```python
from build123d import *

# Parameters (mm, degrees)
F0_W     = 56
F0_H     = 90
F1_DEPTH = 25
F2_DEPTH = 60
F3_SIZE  = 17
F5_D     = 13
F5_DEPTH = 11
F5_TIP   = 3.9055940237
F6_R     = 5


with BuildPart() as f1:
    # F0 (on Top) → F1 (new body)
    with BuildSketch(Plane.XY):
        with Locations((28, 45)):
            Rectangle(F0_W, F0_H)
    extrude(amount=F1_DEPTH)

    # F2 (add): a face of the model
    f2_faces = [f1.faces().sort_by_distance(p)[0] for p in [
        (28, 45, 25),
    ]]
    extrude(f2_faces, amount=F2_DEPTH)

    # F3
    f3_edges = [f1.edges().sort_by_distance(p)[0] for p in [
        (56, 45, 85),
    ]]
    chamfer(f3_edges, length=F3_SIZE)

    # F5
    with Locations(Plane(origin=(62, 0, 62), x_dir=(0, 1, 0), z_dir=(0.7071067812, 0, 0.7071067812))):
        with Locations((20, 20.5269119346), (70, 20.5269119346)):
            Hole(F5_D / 2, depth=F5_DEPTH)
            with Locations((0, 0, -(F5_DEPTH + F5_TIP / 2))):  # 118° drill point
                Cone(0, F5_D / 2, F5_TIP, mode=Mode.SUBTRACT)

    # F6
    f6_edges = [f1.edges().sort_by_distance(p)[0] for p in [
        (28, 0, 0),
        (28, 90, 0),
    ]]
    fillet(f6_edges, radius=F6_R)


solid = f1.part
```
Can you work these out from the model? Positions are in its coordinate system, mm. A direction names the side the tool comes from. Round coordinates to 2 decimals unless told otherwise and drop trailing zeros. Loops run counter-clockwise (first coordinate to the right, second up) from the corner with the lowest first, then second, coordinate; pieces in that order, holes last. Notation, with made-up numbers: M 9,32 L 58,32 A10 cw 58,36 Z; hole C -18,36.5 d9. An arc over 180 degrees is marked long. Answer as a JSON object with one key per item and string values. Group by question number.
Q1. We'd pull the mould along X, two halves only. Please class faces 1 (the flat face through (47, 44, 77)), 2 (the flat face through (0, 44, 42)), 3 (the conical face through (36.75, 20.61, 67.13)), 4 (the cylindrical face through (28, 1, 2)): +X half, -X half, draft (parallel to the pull), parting line (faces both ways), or undercut.
Q2. Please list where these lines run through material, in increasing order: L1, parallel to Y at x = 42.5, z = 73.5; L2, parallel to Y at x = 49, z = 72; L3, parallel to Y at x = 7, z = 4.
Q3. Imagine slicing it at A-A, the plane y = 38. Please give me the cut outline in (x, z), then the cut area to 3 significant figures.
Q4. On a 3-axis mill with a long thin cutter (end or side, diameter ignored), from which of +Z, -Z, +X, -X, +Y, -Y can I reach the whole of each face in a straight line? I mean faces 5 (the conical face through (36.634, 69.853, 67.246)), 6 (the flat face through (28, 46, 0)). Say none if no direction works.
Findings:
{
 "1": {"face 1": "+X half", "face 2": "-X half", "face 3": "undercut", "face 4": "draft"},
 "2": {"L1": "y = 0 to 13.65, 26.35 to 63.65, 76.35 to 90", "L2": "y = 0 to 15.09, 24.91 to 65.09, 74.91 to 90", "L3": "y = 0.1 to 89.9"},
 "3": {"outline": "M 0,0 L 56,0 L 56,68 L 39,85 L 0,85 Z", "area": "4,620 mm2"},
 "4": {"face 5": "none", "face 6": "-Z, +X, -X, +Y, -Y"}
}
